Autodesk Inventor part; units mm, degrees
ref_plane "YZ Plane" through (0, 0, 0) normal (1, 0, 0) x (0, 1, 0)
ref_plane "XZ Plane" through (0, 0, 0) normal (0, 1, 0) x (-1, 0, 0)
ref_plane "XY Plane" through (0, 0, 0) normal (0, 0, 1) x (1, 0, 0)
sketch "Sketch1" plane through (0, 0, 0) normal (0, 1, 0) x (-1, 0, 0)
  line L0 (-28.575, 25.4) -> (28.575, 25.4)
  line L1 (38.1, 15.875) -> (38.1, -15.875)
  line L2 (28.575, -25.4) -> (-28.575, -25.4)
  line L3 (-38.1, -15.875) -> (-38.1, 15.875)
  line L4 (-38.1, 25.4) -> (38.1, -25.4) construction
  line L5 (38.1, 25.4) -> (-38.1, -25.4) construction
  arc A0 (38.1, 15.875) -> (28.575, 25.4) centre (28.575, 15.875) ccw
  arc A1 (-28.575, 25.4) -> (-38.1, 15.875) centre (-28.575, 15.875) ccw
  arc A2 (-38.1, -15.875) -> (-28.575, -25.4) centre (-28.575, -15.875) ccw
  arc A3 (28.575, -25.4) -> (38.1, -15.875) centre (28.575, -15.875) ccw
  line L6 (34.925, -15.875) -> (34.925, 15.875)
  arc A4 (34.925, 15.875) -> (28.575, 22.225) centre (28.575, 15.875) ccw
  line L7 (28.575, 22.225) -> (-28.575, 22.225)
  arc A5 (-28.575, 22.225) -> (-34.925, 15.875) centre (-28.575, 15.875) ccw
  line L8 (-34.925, 15.875) -> (-34.925, -15.875)
  arc A6 (-34.925, -15.875) -> (-28.575, -22.225) centre (-28.575, -15.875) ccw
  line L9 (-28.575, -22.225) -> (28.575, -22.225)
  arc A7 (28.575, -22.225) -> (34.925, -15.875) centre (28.575, -15.875) ccw
  point P0 (0, 0)
  dimension "d0" = 76.2
  dimension "d1" = 50.8
  dimension "d2" = 9.525
  dimension "d3" = 3.175
extrude "Extrusion1" add sketch "Sketch1" along normal blind 1531.1288
sketch "Sketch2" plane through (-28.575, 0, 25.4) normal (0, 0, 1) x (1, 0, 0)
  line L0 (66.675, 0) -> (66.675, 1531.1288)
  line L1 (66.675, 0) -> (-9.525, 216.66)
  line L2 (-9.525, 0) -> (-9.525, 1531.1288)
  line L3 (0, 0) -> (-9.525, 0)
  line L4 (-9.525, 216.66) -> (-9.525, 0)
  line L5 (-9.525, 0) -> (66.675, 0)
  line L6 (66.675, 1531.1288) -> (57.15, 1531.1288)
  line L7 (66.675, 1531.1288) -> (-9.525, 1531.1288)
  line L8 (0, 1531.1288) -> (-9.525, 1531.1288)
  line L9 (-9.525, 1531.1288) -> (-9.525, 1504.329)
  line L10 (-9.525, 1504.329) -> (66.675, 1531.1288)
  point P0 (28.575, 0)
  dimension "d10" = 19.377
  dimension "d12" = 19.377
extrude "Extrusion2" cut sketch "Sketch2" against normal through all contours L5 L3 L2 L1 | L10 L2 L7 L6
equation "\"d0\" = stockWidth"
equation "\"d1\" = stockHeight"
equation "\"d2\" = stockRad"
equation "\"d3\" = stockGuage"
equation "\"d4\" = supSideLen"
equation "\"d10\" = supSideAng"
equation "\"d12\" = supSideAng"
equation "\"height\" = 203.2"
equation "\"shaftDiam\" = 6.35"
equation "\"shaftSpace\" = 1.5875"
equation "\"stageSpace\" = 2.54"
equation "\"stageAngle\" = 15deg"
equation "\"stockHeight\" = 50.8"
equation "\"stockWidth\" = 76.2"
equation "\"stockRad\" = 9.525"
equation "\"stockGuage\" = 3.175"
equation "\"groundActu\" = 304.8"
equation "\"baseWidth\" = 1066.8"
equation "\"baseDepth\" = 254"
equation "\"capThickness\" = 3.175"
equation "\"sup1Len\" = 660.4"
equation "\"sup1Ang\" = 22.619865deg"
equation "\"sup2Len\" = 2079.37366"
equation "\"sup2Ang\" = 8.959949deg"
equation "\"supVertLen\" = 955.13561"
equation "\"supSideLen\" = 1531.12879"
equation "\"supSideAng\" = 19.3769deg"
equation "\"FlangeDiam\" = 12.7"
equation "\"bearingDiam\" = 9.5504"
equation "\"FlangeDepth\" = 1.5875"
equation "\"smallFilet\" = 0.39687"
equation "\"thickness\" = 12.7"
equation "\"ringDiam\" = 96.46608"
properties part number "side support" material "Aluminum 6061"
The listing builds one solid part. Answer for the finished solid, in the listing's coordinates (mm). A direction names the side the tool comes from. Round coordinates to 2 decimals unless told otherwise and drop trailing zeros. Write each loop counter-clockwise with the first axis right and the second up, starting at its lowest first coordinate (ties: lowest second). Pieces come first, ordered by that corner, then holes. Notation, with made-up numbers: M 71.5,-34.75 L 105.5,-34.75 A26 ccw 105.5,-9.75 Z; hole C -26.5,11.25 d6. An arc over 180 degrees is marked long. Write each question's results on one line, items separated by ' | '. Start each with the question number.
Item 1: For a pull along X with two mould halves and no side action, classify faces 3 (the face through (34.925, 759, 0)), 4 (the face through (38.1, 755, 0)), 5 (the face through (-0.178, 1517.666, -22.459)), 6 (the face through (0, 767, 25.4)) as pulls with the +X half, pulls with the -X half, needs draft (parallel to the pull), parting line crosses it, or undercut.
Item 2: A cutting plane is placed at A-A on z = 5. Write down the section's boundary in (x, y) (1 decimal), and give its area (3 significant figures).
Item 3: Straight lines are drawn through the part: L1, parallel to X at y = 1385, z = 1 (3 decimals); L2, parallel to Z at x = -28.5, y = 957 (3 decimals); L3, parallel to X at y = 1165.5, z = 17.5. For each, find the intervals that lie inside material, in ascending order. Write a range as [from, to].
Item 4: For faces 1 (the face through (0, 767, 22.225)), 2 (the face through (-38.1, 851, 0)), determine the directions among +Z, -Z, +X, -X, +Y, -Y from which every point of the face is accessible in a straight line to the end or side of a thin tool.
Item 5: A cutting plane is placed at C-C on y = 1368. Write down the section's boundary in (x, z) (3 decimals), and give its area (3 significant figures).
Item 6: A cutting plane is placed at B-B on x = 8. Write down the section's boundary in (y, z) (3 decimals), and give its area (3 significant figures).
Item 7: A flat-ended cylindrical pin translates along its axis: pin 1 Ø10 at (x, z) = (5, -14.5) entering from +Y. Find the tip coordinate at first contact, or state that the pin passes through.
Check sheet entries:
1) face 3: undercut | face 4: pulls with the +X half | face 5: pulls with the -X half | face 6: needs draft
2) outline: M -38.1,216.7 L -34.9,207.6 L -34.9,1505.4 L -38.1,1504.3 Z; M 34.9,9 L 38.1,0 L 38.1,1531.1 L 34.9,1530 Z | area: 8,950 mm²
3) L1: [-38.1, -34.925], [34.925, 38.1] | L2: [-25.4, -22.225], [22.225, 25.4] | L3: [-37.96, -34.71], [34.71, 37.96]
4) face 1: +Y, -Y | face 2: +Z, -Z, -X, +Y, -Y
5) outline: M -38.1,-15.875 A9.525 ccw -28.575,-25.4 L 28.575,-25.4 A9.525 ccw 38.1,-15.875 L 38.1,15.875 A9.525 ccw 28.575,25.4 L -28.575,25.4 A9.525 ccw -38.1,15.875 Z; hole M -34.925,-15.875 A6.35 ccw -28.575,-22.225 L 28.575,-22.225 A6.35 ccw 34.925,-15.875 L 34.925,15.875 A6.35 ccw 28.575,22.225 L -28.575,22.225 A6.35 ccw -34.925,15.875 Z | area: 723 mm²
6) outline: M 85.584,-25.4 L 1520.543,-25.4 L 1520.543,-22.225 L 85.584,-22.225 Z; M 85.584,22.225 L 1520.543,22.225 L 1520.543,25.4 L 85.584,25.4 Z | area: 9,110 mm²
7) pin 1: through
